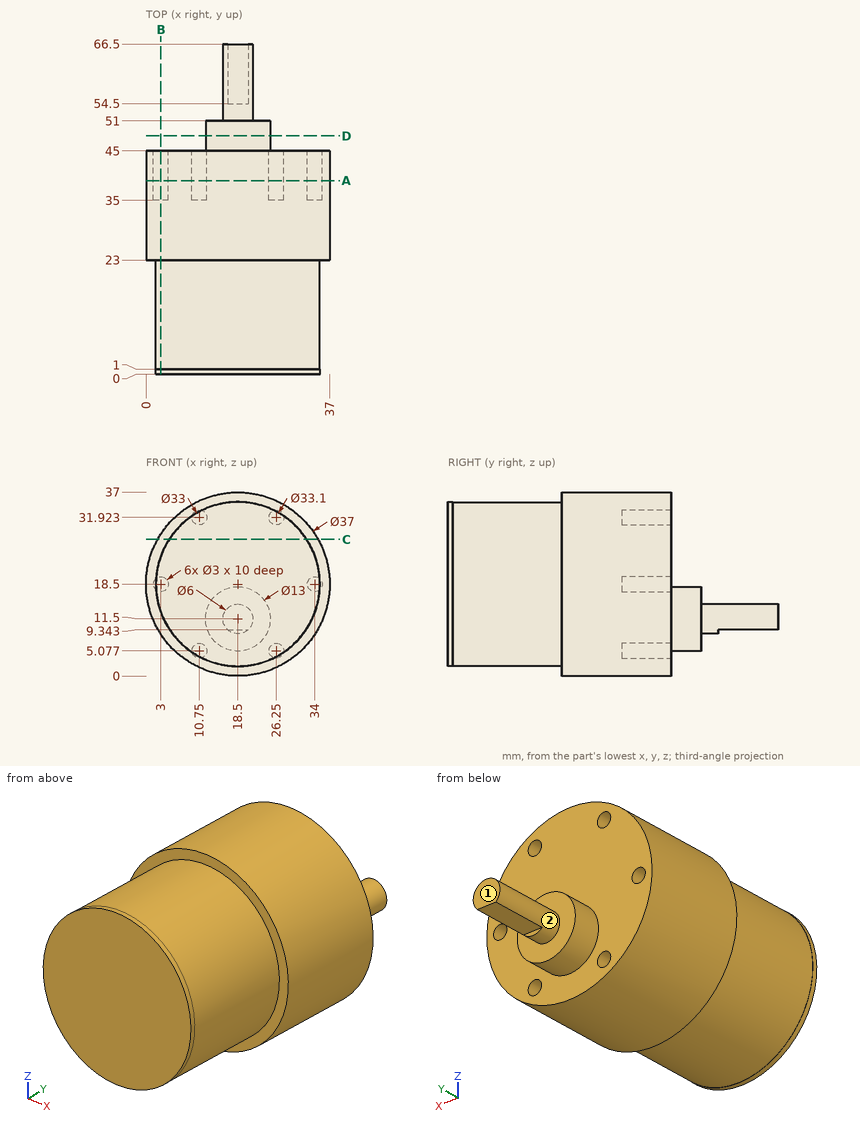
Check sheet for the drawn part. Datum: minimum x, y, z corner. Units: mm. A direction names the side the tool comes from. Give positions to 0.01 mm unless a question says otherwise; leave off trailing zeros. Order: outer loops, then holes, each group sorted by start corner. A loop starts at its lowest first (then second) coordinate and runs counter-clockwise, first axis right, second up. Notation, with made-up numbers: (64.5, 3.25) - (95.5, 3.25) arc R26 ccw to (95.5, 24.25) - close; hole circle Ø4 at (-29.75, 35.5). An arc over 180 degrees is marked (long way). Write item = value, one per line. Start each with the question number.
1) Section check D-D (y = 48). Enter the section's corners in (x, z), then the cut area to 3 significant figures.
2) Access from +Z, -Z, +X, -X, +Y, -Y to the whole of each face (thin tool, end or side, straight path). Record for the marked faces 1 and 2.
3) Section check C-C (z = 27.5). Enter the section's corners in (x, y), then the cut area to 3 significant figures.
4) Scan lines: L1, parallel to X at y = 40, z = 18 (1 decimal); L2, parallel to Z at x = 10, y = 38 (1 decimal); L3, parallel to Y at x = 16, z = 6. Record each from-to range of solid material in increasing order.
5) Gauge pin test, flat ends, axial feed: pin 1 Ø2.5 at (x, z) = (3, 18.5) entering from +Y; pin 2 Ø3.5 at (x, z) = (10.75, 31.92) entering from -Y; pin 3 Ø2 at (x, z) = (12, 26) entering from +Y; pin 4 Ø6 at (x, y) = (28, 12.5) entering from +Z (1 decimal). Record the tip position at first contact, or that the pin passes through.
6) Section check B-B (x = 3). Enter the section's corners in (y, z), then the cut area to 3 significant figures.
7) Section check A-A (y = 39). Enter the section's corners in (x, z), then the cut area to 3 significant figures.
Geometry check:
q1.outline = circle Ø13 at (18.5, 11.5)
q1.area = 133 mm2
q2.face_1 = +Z, -Z, +X, -X, +Y
q2.face_2 = +Y
q3.outline = (2.34, 23) - (4.67, 23) - (4.67, 1) - (4.61, 1) - (4.61, 0) - (32.39, 0) - (32.39, 1) - (32.33, 1) - (32.33, 23) - (34.66, 23) - (34.66, 45) - (2.34, 45) - close
q3.area = 1,350 mm2
q4.L1 = 0 to 1.6, 4.4 to 32.6, 35.4 to 37
q4.L2 = 2.1 to 3.8, 6.4 to 30.6, 33.2 to 34.9
q4.L3 = 0 to 51
q5.pin_1 = 35
q5.pin_2 = 0
q5.pin_3 = 45
q5.pin_4 = 33.7
q6.outline = (0, 12.7) - (1, 12.7) - (1, 12.84) - (23, 12.84) - (23, 8.4) - (45, 8.4) - (45, 17) - (35, 17) - (35, 20) - (45, 20) - (45, 28.6) - (23, 28.6) - (23, 24.16) - (1, 24.16) - (1, 24.3) - (0, 24.3) - close
q6.area = 675 mm2
q7.outline = circle Ø37 at (18.5, 18.5); hole circle Ø3 at (3, 18.5); hole circle Ø3 at (10.75, 5.08); hole circle Ø3 at (10.75, 31.92); hole circle Ø3 at (26.25, 5.08); hole circle Ø3 at (26.25, 31.92); hole circle Ø3 at (34, 18.5)
q7.area = 1,030 mm2
